Model file for the job. Use its own axes, mm. A direction names the side the tool comes from. Give positions to 0.01 mm unless a question says otherwise; leave off trailing zeros. Write each loop counter-clockwise with the first axis right and the second up, starting at its lowest first coordinate (ties: lowest second). Pieces come first, ordered by that corner, then holes.
```python
from build123d import *

# Parameters (mm, degrees)
SKETCH1_W                        = 25
SKETCH1_H                        = 7
BOSS_EXTRUDE1_DEPTH              = 65
SKETCH2_W                        = 11
SKETCH2_H                        = 8
CUT_EXTRUDE1_DEPTH               = 67.560123197
CHAMFER1_SIZE                    = 1
CBORE_FOR_M2_5_SHCS2_D           = 2.9
CBORE_FOR_M2_5_SHCS2_CBORE_D     = 5.5
CBORE_FOR_M2_5_SHCS2_CBORE_DEPTH = 2.5
FILLET1_R                        = 2
CHAMFER2_SIZE                    = 1
SKETCH10_W                       = 25
SKETCH10_H                       = 4
CUT_EXTRUDE2_DEPTH               = 10
FILLET2_R                        = 1


with BuildPart() as part:
    # Sketch1 → Boss-Extrude1 (new body)
    with BuildSketch(Plane.XY):
        Rectangle(SKETCH1_W, SKETCH1_H)
    extrude(amount=BOSS_EXTRUDE1_DEPTH)

    # Sketch2 → Cut-Extrude1 (cut, through all)
    with BuildSketch(Plane(origin=(0, 3.5, 0), x_dir=(1, 0, 0), z_dir=(0, 1, 0))):
        with Locations((0, -61)):
            Rectangle(SKETCH2_W, SKETCH2_H)
    extrude(amount=-CUT_EXTRUDE1_DEPTH, mode=Mode.SUBTRACT)

    # Chamfer1
    chamfer1_edges = [part.edges().sort_by_distance(p)[0] for p in [
        (-5.5, 0, 57),
        (5.5, 0, 57),
    ]]
    chamfer(chamfer1_edges, length=CHAMFER1_SIZE)

    # CBORE for M2.5 SHCS2 (through all)
    with Locations(Plane(origin=(12.5, -6.575007997, 116.706532938), x_dir=(0, 0, -1), z_dir=(1, 0, 0))):
        with Locations((55.706532938, 6.575007997)):
            CounterBoreHole(CBORE_FOR_M2_5_SHCS2_D / 2, CBORE_FOR_M2_5_SHCS2_CBORE_D / 2, CBORE_FOR_M2_5_SHCS2_CBORE_DEPTH)

    # Fillet1
    # the kernel refuses this fillet: 2 mm, written as the material it takes off along each edge
    with BuildSketch(Plane(origin=(12.5, -3.5, -5), x_dir=(-1, 0, 0), z_dir=(0, 0, 1)), Plane(origin=(12.5, 3.5, -5), x_dir=(0, -1, 0), z_dir=(0, 0, 1))) as fillet1_piece_1:
        with BuildLine():
            CenterArc((FILLET1_R, -FILLET1_R), FILLET1_R, 90, 90)
            Line((0, -FILLET1_R), (0, 0))
            Line((0, 0), (FILLET1_R, 0))
        make_face()
    extrude(amount=75, mode=Mode.SUBTRACT)
    with BuildSketch(Plane(origin=(-12.5, -3.5, -5), x_dir=(1, 0, 0), z_dir=(0, 0, 1)), Plane(origin=(-12.5, 3.5, -5), x_dir=(0, -1, 0), z_dir=(0, 0, 1))) as fillet1_piece_2:
        with BuildLine():
            CenterArc((FILLET1_R, FILLET1_R), FILLET1_R, 180, 90)
            Line((0, FILLET1_R), (0, 0))
            Line((0, 0), (FILLET1_R, 0))
        make_face()
    extrude(amount=75, mode=Mode.SUBTRACT)

    # Chamfer2
    chamfer2_edges = [part.edges().sort_by_distance(p)[0] for p in [
        (-5.5, 0, 65),
        (5.5, 0, 65),
    ]]
    chamfer(chamfer2_edges, length=CHAMFER2_SIZE)

    # Sketch10 → Cut-Extrude2 (cut)
    with BuildSketch(Plane(origin=(0, 0, 0), x_dir=(-1, 0, 0), z_dir=(0, 0, -1))):
        with Locations((0, -1.5)):
            Rectangle(SKETCH10_W, SKETCH10_H)
    extrude(amount=-CUT_EXTRUDE2_DEPTH, mode=Mode.SUBTRACT)

    # Fillet2
    fillet2_edges = [part.edges().sort_by_distance(p)[0] for p in [
        (0, 0.5, 10),
    ]]
    fillet(fillet2_edges, radius=FILLET2_R)


solid = part.part
```
1. Pull direction X, two halves, no side cores. Call faces 1 (the flat face through (12.5, 0, 64)), 2 (the flat face through (0, 0.5, 4)), 3 (the flat face through (-5.5, 0.8, 62.4)): +X half, -X half, draft (parallel to the pull), parting line (faces both ways), or undercut.
Calculated:
face 1: +X half
face 2: draft
face 3: undercut
2. Which spindle directions (+Z, -Z, +X, -X, +Y, -Y) get a long thin tool onto all of the face, cutting with end or side? Do faces 4 (the flat face through (5.5, 0.8, 62.4)), 5 (the cylindrical face through (11.268, -2.685, 61.596)), 6 (the flat face through (0, -3.5, 37)). Say none if no direction does.
Calculated:
face 4: +Z, +Y, -Y
face 5: +X
face 6: +Z, -Z, +X, -X, -Y
3. Probe probe 1 along Y at (x, z) = (-8.5, 61); probe 2 along Z at (x, y) = (0, -1.25); probe 3 along Y at (x, z) = (10.85, 61). List the from-to ranges inside material, lowest first.
Calculated:
probe 1: y = -3.5 to -1.45, 1.45 to 3.5
probe 2: z = 10 to 57
probe 3: y = -3.47 to -2.75, 2.75 to 3.47
4. Slice it at C-C, the plane z = 61. Write the cut outline in (x, y).
Calculated:
outline: (-12.5, -1.5) arc R2 ccw to (-10.5, -3.5) - (-5.5, -3.5) - (-5.5, -1.45) - (-12.5, -1.45) - close; (-12.5, 1.45) - (-5.5, 1.45) - (-5.5, 3.5) - (-10.5, 3.5) arc R2 ccw to (-12.5, 1.5) - close; (5.5, -3.5) - (10.5, -3.5) arc R2 ccw to (12.06, -2.75) - (10, -2.75) - (10, -1.45) - (5.5, -1.45) - close; (5.5, 1.45) - (10, 1.45) - (10, 2.75) - (12.06, 2.75) arc R2 ccw to (10.5, 3.5) - (5.5, 3.5) - close
5. Pin check, flat tips, straight feed: P1, Ø4.5, axis at x = 5.5, z = 5.5, coming from the -Y side; P2, Ø1.5, axis at x = -3.5, y = -1.5, coming from the -Z side; P3, Ø3.5, axis at y = 0, z = 61, coming from the +X side. Stop position of each tip, or through.
Calculated:
P1: stops at y = 0.5
P2: stops at z = 10
P3: stops at x = 10
6. Slice it at B-B, the plane z = 45.5. Write the cut outline in (x, y).
Calculated:
outline: (-12.5, -1.5) arc R2 ccw to (-10.5, -3.5) - (10.5, -3.5) arc R2 ccw to (12.5, -1.5) - (12.5, 1.5) arc R2 ccw to (10.5, 3.5) - (-10.5, 3.5) arc R2 ccw to (-12.5, 1.5) - close
7. Slice it at A-A, the plane x = -1. Write the cut outline in (y, z), and give its area (3 significant figures).
Calculated:
outline: (-3.5, 10) - (-0.5, 10) arc R1 cw to (0.5, 9) - (0.5, 0) - (3.5, 0) - (3.5, 57) - (-3.5, 57) - close
area: 359 mm2
